```python
from build123d import *

# Parameters (mm, degrees)
F1_DEPTH = 5
F2_D     = 2.5
F2_DEPTH = 15
F2_TIP   = 0.7510757738
F3_SIZE  = 4


with BuildPart() as f1:
    # F0 (on Front) → F1 (new body)
    with BuildSketch(Plane.XZ):
        with BuildLine():
            Line((39.9999981374, 27.0838558645), (-40.0000018626, 27.0838558645))
            ThreePointArc((-40.0000018626, 27.0838558645), (-43.5355357686, 25.6193897704), (-45.0000018626, 22.0838558645))
            Line((-45.0000018626, 22.0838558645), (-45.0000018626, 12.0838558645))
            Line((-45.0000018626, 12.0838558645), (-37.5000018626, 12.0838558645))
            Line((-37.5000018626, 12.0838558645), (37.4999981374, 12.0838558645))
            Line((37.4999981374, 12.0838558645), (44.9999981374, 12.0838558645))
            Line((44.9999981374, 12.0838558645), (44.9999981374, 22.0838558645))
            ThreePointArc((44.9999981374, 22.0838558645), (43.5355320433, 25.6193897704), (39.9999981374, 27.0838558645))
        make_face()
        with BuildLine():
            Line((-37.5000018626, 12.0838558645), (-45.0000018626, 12.0838558645))
            Line((-45.0000018626, 12.0838558645), (-45.0000018626, 2.0838558645))
            ThreePointArc((-45.0000018626, 2.0838558645), (-43.5355357686, -1.4516780414), (-40.0000018626, -2.9161441355))
            Line((-40.0000018626, -2.9161441355), (39.9999981374, -2.9161441355))
            ThreePointArc((39.9999981374, -2.9161441355), (43.5355320433, -1.4516780414), (44.9999981374, 2.0838558645))
            Line((44.9999981374, 2.0838558645), (44.9999981374, 12.0838558645))
            Line((44.9999981374, 12.0838558645), (37.4999981374, 12.0838558645))
            Line((37.4999981374, 12.0838558645), (-37.5000018626, 12.0838558645))
        make_face()
    extrude(amount=F1_DEPTH)

    # F2
    with Locations(Plane(origin=(0, 0, 0), x_dir=(1, 0, 0), z_dir=(0, 1, 0))):
        with Locations((-37.5000018626, -12.0838558645), (37.4999981374, -12.0838558645)):
            Hole(F2_D / 2, depth=F2_DEPTH)
            with Locations((0, 0, -(F2_DEPTH + F2_TIP / 2))):  # 118° drill point
                Cone(0, F2_D / 2, F2_TIP, mode=Mode.SUBTRACT)

    # F3
    f3_edges = [f1.edges().sort_by_distance(p)[0] for p in [
        (-2e-06, 0, -2.916144),
    ]]
    chamfer(f3_edges, length=F3_SIZE)


solid = f1.part
```
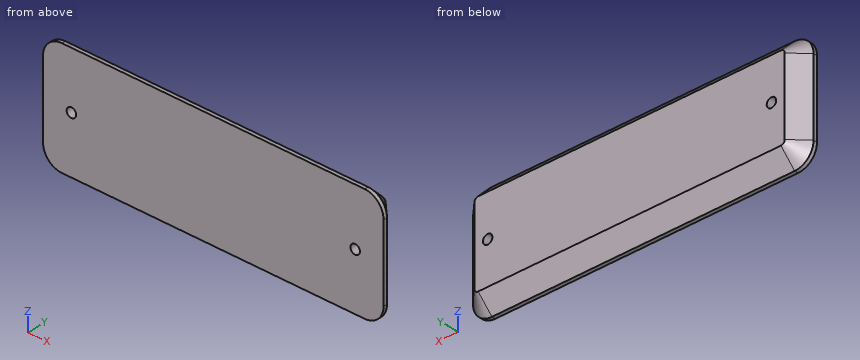
Geometry check sheet. Reference: the model listing, model coordinates, mm. Give positions to 0.01 mm unless a question says otherwise; leave off trailing zeros. Write each loop counter-clockwise with the first axis right and the second up, starting at its lowest first coordinate (ties: lowest second). Pieces come first, ordered by that corner, then holes. Notation, with made-up numbers: (61.25, 26.25) - (99.25, 26.25) arc R23 cw to (99.25, 65.25) - close; hole circle Ø7 at (62, 12). An arc over 180 degrees is marked (long way). Use a Markdown table: item, result.
Q1. Section check C-C, the plane z = 16.5. Enter the section's corners in (x, y), then the cut area to 3 significant figures.
Computed:
| item | result |
|---|---|
| outline | (-45, -5) - (45, -5) - (45, -4) - (41, 0) - (-41, 0) - (-45, -4) - close |
| area | 434 mm² |
Q2. Section check B-B, the plane x = 3. Enter the section's corners in (y, z), then the cut area to 3 significant figures.
Computed:
| item | result |
|---|---|
| outline | (-5, -2.92) - (-4, -2.92) - (0, 1.08) - (0, 23.08) - (-4, 27.08) - (-5, 27.08) - close |
| area | 134 mm² |
Q3. Thickness scan on L1, parallel to Z at x = 37.5, y = -4.2; L2, parallel to X at y = -1.4, z = 12; L3, parallel to X at y = -4.3, z = 2. Record the ranges inside material, lowest first. Write a range as [from, to].
Computed:
| item | result |
|---|---|
| L1 | z = [-2.92, 10.83], [13.33, 27.08] |
| L2 | x = [-42.4, -38.75], [-36.25, 36.25], [38.75, 42.4] |
| L3 | x = [-45, 45] |
Q4. Go/stop test with flat-tipped pins: P1, Ø2, axis at x = 37.5, z = 12.08, coming from the +Y side; P2, Ø1.5, axis at x = -9, y = -2, coming from the +Z side; P3, Ø2, axis at y = -1, z = 18, coming from the -X side. Record where each tip stops, or that it passes through.
Computed:
| item | result |
|---|---|
| P1 | passes through |
| P2 | stops at z = 25.83 |
| P3 | stops at x = -43 |
Q5. Section check A-A, the plane y = -1.15. Enter the section's corners in (x, z), then the cut area to 3 significant figures.
Computed:
| item | result |
|---|---|
| outline | (-42.15, 2.08) arc R2.15 ccw to (-40, -0.07) - (40, -0.07) arc R2.15 ccw to (42.15, 2.08) - (42.15, 22.08) arc R2.15 ccw to (40, 24.23) - (-40, 24.23) arc R2.15 ccw to (-42.15, 22.08) - close; hole circle Ø2.5 at (-37.5, 12.08); hole circle Ø2.5 at (37.5, 12.08) |
| area | 2,030 mm² |
